from build123d import *

# Parameters (mm, degrees)
ESBO_O1_W                = 17
ESBO_O1_H                = 14.6
RESSALTO_EXTRUS_O1_DEPTH = 1.2
ESBO_O2_R                = 2
ESBO_O2_R_2              = 2.054882152
CORTE_EXTRUS_O3_DEPTH    = 18.446203025
RESSALTO_EXTRUS_O4_DEPTH = 9
ESBO_O8_R                = 1.15
CORTE_EXTRUS_O4_DEPTH    = 3
ESBO_O10_W               = 8
ESBO_O10_H               = 2.5
RESSALTO_EXTRUS_O5_DEPTH = 7
ESBO_O11_R               = 1.5
CORTE_EXTRUS_O5_DEPTH    = 10
CORTE_EXTRUS_O8_DEPTH    = 9
FILETE1_R                = 3
FILETE2_R                = 3


with BuildPart() as part:
    # Esboço1 → Ressalto-extrusão1 (new body)
    with BuildSketch(Plane(origin=(0, 0, 0), x_dir=(1, 0, 0), z_dir=(0, 1, 0))):
        Rectangle(ESBO_O1_W, ESBO_O1_H)
        Polygon((-15.8, 0), (-8.5, 7.3), (-8.5, -7.3), align=None)
        Polygon((8.5, -7.3), (15.8, 0), (8.5, 7.3), align=None)
    extrude(amount=RESSALTO_EXTRUS_O1_DEPTH)

    # Esboço2 → Corte-extrusão3 (cut, through all)
    with BuildSketch(Plane(origin=(0, 1.2, 0), x_dir=(1, 0, 0), z_dir=(0, 1, 0))):
        with Locations(Location((-9.75, 0.5, 0), (0, 0, 270))):
            Circle(ESBO_O2_R)
        with Locations(Location((0, 3.5, 0), (0, 0, 270))):
            Circle(ESBO_O2_R_2)
        with Locations(Location((9.75, 0.5, 0), (0, 0, 270))):
            Circle(ESBO_O2_R)
    extrude(amount=-CORTE_EXTRUS_O3_DEPTH, mode=Mode.SUBTRACT)

    # Esboço6 → Ressalto-extrusão4 (add)
    with BuildSketch(Plane(origin=(0, 1.2, 0), x_dir=(1, 0, 0), z_dir=(0, 1, 0))):
        Polygon((-14.3, -1.5), (14.3, -1.5), (8.5, -7.3), (-8.5, -7.3), align=None)
    extrude(amount=RESSALTO_EXTRUS_O4_DEPTH)

    # Esboço8 → Corte-extrusão4 (cut)
    with BuildSketch(Plane(origin=(0, 0, 1.5), x_dir=(-1, 0, 0), z_dir=(0, 0, -1))):
        with Locations((-9.8, 6.7)):
            Circle(ESBO_O8_R)
        with Locations((9.75, 6.7)):
            Circle(ESBO_O8_R)
    extrude(amount=-CORTE_EXTRUS_O4_DEPTH, mode=Mode.SUBTRACT)

    # Esboço10 → Ressalto-extrusão5 (add)
    with BuildSketch(Plane(origin=(0, 10.2, 0), x_dir=(1, 0, 0), z_dir=(0, 1, 0))):
        with Locations((0, -6.05)):
            Rectangle(ESBO_O10_W, ESBO_O10_H)
    extrude(amount=RESSALTO_EXTRUS_O5_DEPTH)

    # Esboço11 → Corte-extrusão5 (cut)
    with BuildSketch(Plane(origin=(0, 0, 4.8), x_dir=(-1, 0, 0), z_dir=(0, 0, -1))):
        with Locations((0, 13.8)):
            Circle(ESBO_O11_R)
    extrude(amount=-CORTE_EXTRUS_O5_DEPTH, mode=Mode.SUBTRACT)

    # Esboço12 → Corte-extrusão8 (cut)
    with BuildSketch(Plane(origin=(0, 10.2, 0), x_dir=(1, 0, 0), z_dir=(0, 1, 0))):
        Polygon((-3.957764838, -3.75), (-5.8, -1.5), (5.8, -1.5), (3.98902582, -3.75), align=None)
    extrude(amount=-CORTE_EXTRUS_O8_DEPTH, mode=Mode.SUBTRACT)

    # Filete1
    filete1_edges = [part.edges().sort_by_distance(p)[0] for p in [
        (4, 17.2, 6.05),
    ]]
    fillet(filete1_edges, radius=FILETE1_R)

    # Filete2
    filete2_edges = [part.edges().sort_by_distance(p)[0] for p in [
        (-4, 17.2, 6.05),
    ]]
    fillet(filete2_edges, radius=FILETE2_R)


solid = part.part
Verification items for the finished model (mm, model axes). A direction names the side the tool comes from. Round coordinates to 2 decimals unless told otherwise and drop trailing zeros. Loops run counter-clockwise (first coordinate to the right, second up) from the corner with the lowest first, then second, coordinate; pieces in that order, holes last. Notation, with made-up numbers: (24, 6) - (75, 6) arc R28 cw to (75, 42) - close; hole circle Ø4 at (-10, 75.5). An arc over 180 degrees is marked (long way). Use a Markdown table: item, result. Add a question column.
1. Section check B-B, the plane y = 6.7. Record the boundary of the cut face in (x, z).
2. Gauge pin test, flat ends, axial feed: pin 1 (4 mm diameter, centred on x = -11.5, y = 7.5, fed in from -Z); pin 2 (3.5 mm diameter, centred on x = -1, y = 14, fed in from -Z); pin 3 (3 mm diameter, centred on x = -2, z = 2.5, fed in from +Y). Record the tip position at first contact, or that the pin passes through.
3. Section check A-A, the plane x = 0. Record the boundary of the cut face in (y, z), plus the area to 3 significant figures.
4. Thickness scan on probe 1 along X at (y, z) = (6.5, 3.5); probe 2 along X at (y, z) = (0.9, -0.5); probe 3 along Y at (x, z) = (0, 6.1). Record the ranges inside material, lowest first. Write a range as [from, to].
5. Section check C-C, the plane z = -0.5. Record the boundary of the cut face in (x, y), plus the area to 3 significant figures.
6. Section check D-D, the plane z = 5.75. Record the boundary of the cut face in (x, y).
7. Release check for a two-part mould opening along X. For faces 5 (the face through (11.4, 5, 4.4)), 6 (the face through (10, 5, 1.5)), 7 (the face through (-10, 7, 4.5)), 8 (the face through (-3.1, 16.34, 6.03)) record: released by +X, released by -X, zero draft, split by the parting line, or undercut.
8. Access from +Z, -Z, +X, -X, +Y, -Y to the whole of each face (thin tool, end or side, straight path). Record for faces 1 (the face through (-10, 5, 1.5)), 2 (the face through (-7.767, 0.608, -0.76)), 3 (the face through (10.95, 6.75, 2.98)), 4 (the face through (4.907, 5.763, 2.609)).
Checks:
| question | item | result |
|---|---|---|
| 1 | outline | (-14.3, 1.5) - (-10.9, 1.5) - (-10.9, 4.5) - (-8.6, 4.5) - (-8.6, 1.5) - (-5.8, 1.5) - (-3.96, 3.75) - (3.99, 3.75) - (5.8, 1.5) - (8.65, 1.5) - (8.65, 4.5) - (10.95, 4.5) - (10.95, 1.5) - (14.3, 1.5) - (8.5, 7.3) - (-8.5, 7.3) - close |
| 2 | pin 1 | stops at z = 1.5 |
| 2 | pin 2 | stops at z = 4.8 |
| 2 | pin 3 | stops at y = 10.2 |
| 3 | outline | (0, -7.3) - (1.2, -7.3) - (1.2, -5.55) - (0, -5.55) - close; (0, -1.45) - (1.2, -1.45) - (1.2, 3.75) - (10.2, 3.75) - (10.2, 4.8) - (12.3, 4.8) - (12.3, 7.3) - (0, 7.3) - close; (15.3, 4.8) - (17.2, 4.8) - (17.2, 7.3) - (15.3, 7.3) - close |
| 3 | area | 54.5 mm^2 |
| 4 | probe 1 | x = [-12.3, -10.88], [-8.62, -4.16], [4.19, 8.67], [10.93, 12.3] |
| 4 | probe 2 | x = [-15.3, -11.75], [-7.75, 7.75], [11.75, 15.3] |
| 4 | probe 3 | y = [0, 12.3], [15.3, 17.2] |
| 5 | outline | (-15.3, 0) - (-11.75, 0) - (-11.75, 1.2) - (-15.3, 1.2) - close; (-7.75, 0) - (7.75, 0) - (7.75, 1.2) - (-7.75, 1.2) - close; (11.75, 0) - (15.3, 0) - (15.3, 1.2) - (11.75, 1.2) - close |
| 5 | area | 27.1 mm^2 |
| 6 | outline | (-10.05, 0) - (10.05, 0) - (10.05, 10.2) - (4, 10.2) - (4, 14.2) arc R3 ccw to (1, 17.2) - (-1, 17.2) arc R3 ccw to (-4, 14.2) - (-4, 10.2) - (-10.05, 10.2) - close; hole circle Ø3 at (0, 13.8) |
| 7 | face 5 | released by +X |
| 7 | face 6 | zero draft |
| 7 | face 7 | undercut |
| 7 | face 8 | released by -X |
| 8 | face 1 | -Z, +X, -X, +Y |
| 8 | face 2 | +Y, -Y |
| 8 | face 3 | -Z |
| 8 | face 4 | -Z, +Y |
